Check sheet for the modelled part. Datum: model origin and axes. Units: mm. Round coordinates to 2 decimals unless told otherwise and drop trailing zeros. Write each loop counter-clockwise with the first axis right and the second up, starting at its lowest first coordinate (ties: lowest second). Pieces come first, ordered by that corner, then holes. Notation, with made-up numbers: M 3.25,35.5 L 18.25,35.5 A29 ccw 18.25,61.5 Z; hole C -6,40.5 d10. An arc over 180 degrees is marked long. Answer in a Markdown table with one row per item.
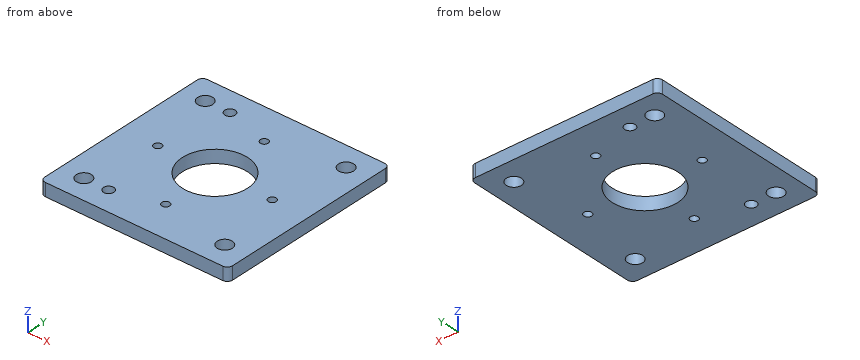
```python
from build123d import *

# Parameters (mm, degrees)
SKETCH1_W           = 72
SKETCH1_H           = 72
SKETCH1_R           = 2.9
SKETCH1_R_2         = 12.5
SKETCH1_R_3         = 1.5
SKETCH1_R_4         = 2
BOSS_EXTRUDE1_DEPTH = 5
FILLET1_R           = 2


with BuildPart() as part:
    # Sketch1 → Boss-Extrude1 (new body)
    with BuildSketch(Plane.XY):
        Rectangle(SKETCH1_W, SKETCH1_H)
        with Locations((-27, 27)):
            Circle(SKETCH1_R, mode=Mode.SUBTRACT)
        with Locations((27, 27)):
            Circle(SKETCH1_R, mode=Mode.SUBTRACT)
        with Locations((27, -27)):
            Circle(SKETCH1_R, mode=Mode.SUBTRACT)
        with Locations((-27, -27)):
            Circle(SKETCH1_R, mode=Mode.SUBTRACT)
        Circle(SKETCH1_R_2, mode=Mode.SUBTRACT)
        with Locations((0, 21.92)):
            Circle(SKETCH1_R_3, mode=Mode.SUBTRACT)
        with Locations((0, -21.92)):
            Circle(SKETCH1_R_3, mode=Mode.SUBTRACT)
        with Locations((-21.92, 0)):
            Circle(SKETCH1_R_3, mode=Mode.SUBTRACT)
        with Locations((21.92, 0)):
            Circle(SKETCH1_R_3, mode=Mode.SUBTRACT)
        with Locations((-17.5, 27)):
            Circle(SKETCH1_R_4, mode=Mode.SUBTRACT)
        with Locations((-17.5, -27)):
            Circle(SKETCH1_R_4, mode=Mode.SUBTRACT)
    extrude(amount=BOSS_EXTRUDE1_DEPTH)

    # Fillet1
    fillet1_edges = [part.edges().sort_by_distance(p)[0] for p in [
        (-36, 36, 2.5),
        (36, 36, 2.5),
        (36, -36, 2.5),
        (-36, -36, 2.5),
    ]]
    fillet(fillet1_edges, radius=FILLET1_R)


solid = part.part
```
1. Go/stop test with a flat-tipped pin: pin 1 (3.5 mm diameter, centred on x = -17.5, y = -27, fed in from -Z). Record where the tip stops, or that it passes through.
Found:
| item | result |
|---|---|
| pin 1 | passes through |
2. Section check A-A, the plane y = 27. Record the cut outline in (x, z), and give its area (3 significant figures).
Found:
| item | result |
|---|---|
| outline | M -36,0 L -29.9,0 L -29.9,5 L -36,5 Z; M -24.1,0 L -19.5,0 L -19.5,5 L -24.1,5 Z; M -15.5,0 L 24.1,0 L 24.1,5 L -15.5,5 Z; M 29.9,0 L 36,0 L 36,5 L 29.9,5 Z |
| area | 282 mm2 |
3. Scan lines: L1, parallel to Y at x = 0, z = 2.4; L2, parallel to Y at x = 27, z = 2.35; L3, parallel to X at y = -27.5, z = 1.45. Record each from-to range of solid material in increasing order.
Found:
| item | result |
|---|---|
| L1 | y = -36 to -23.42, -20.42 to -12.5, 12.5 to 20.42, 23.42 to 36 |
| L2 | y = -36 to -29.9, -24.1 to 24.1, 29.9 to 36 |
| L3 | x = -36 to -29.86, -24.14 to -19.44, -15.56 to 24.14, 29.86 to 36 |
4. Section check D-D, the plane x = 10.5. Record the cut outline in (y, z).
Found:
| item | result |
|---|---|
| outline | M -36,0 L -6.78,0 L -6.78,5 L -36,5 Z; M 6.78,0 L 36,0 L 36,5 L 6.78,5 Z |
5. Section check C-C, the plane z = 3.65. Count the separate pieces of the cut face and the enclosed holes in it, and give its area (3 significant figures).
Found:
| item | result |
|---|---|
| separate pieces | 1 |
| enclosed holes | 11 |
| area | 4,530 mm2 |
6. Section check B-B, the plane x = 27. Record the cut outline in (y, z), and give its area (3 significant figures).
Found:
| item | result |
|---|---|
| outline | M -36,0 L -29.9,0 L -29.9,5 L -36,5 Z; M -24.1,0 L 24.1,0 L 24.1,5 L -24.1,5 Z; M 29.9,0 L 36,0 L 36,5 L 29.9,5 Z |
| area | 302 mm2 |
